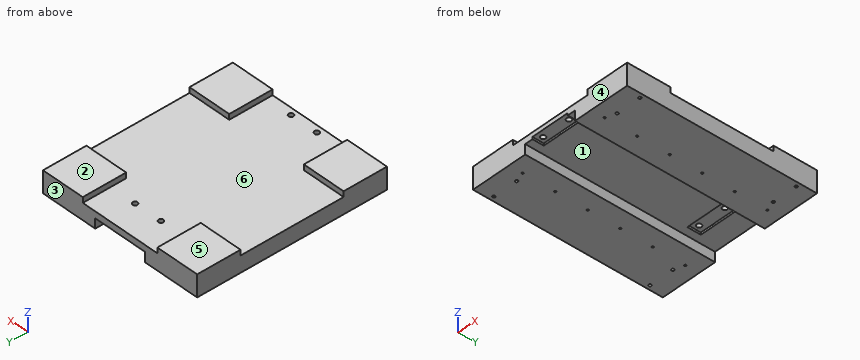
```python
from build123d import *

# Parameters (mm, degrees)
SKETCH_1_W                  = 310
SKETCH_1_H                  = 350
EXTRUDE_1_DEPTH             = 30
SKETCH_2_W                  = 100
SKETCH_2_H                  = 18
CUT_EXTRUDE_1_DEPTH         = 384.959633295
SKETCH_3_W                  = 80
SKETCH_3_H                  = 80
EXTRUDE_2_DEPTH             = 10
SKETCH_5_W                  = 71
SKETCH_5_H                  = 4
CUT_EXTRUDE_3_DEPTH         = 21
SKETCH_7_W                  = 71
SKETCH_7_H                  = 25
CUT_EXTRUDE_4_DEPTH         = 4
SKETCH_8_R                  = 4.5
CUT_EXTRUDE_5_DEPTH         = 235.806303152
HOLE_WIZARD_M6_1_D          = 5
HOLE_WIZARD_M6_1_DEPTH      = 12
HOLE_WIZARD_M6_1_TIP        = 1.502151548
HOLE_WIZARD_M4_1_AT_2_COUNT = 2
HOLE_WIZARD_M4_1_AT_2_PITCH = 165
PATTERN_LINEAR_1_COUNT      = 6
PATTERN_LINEAR_1_PITCH      = 60


with BuildPart() as part:
    # 草图1 → 凸台-拉伸1 (new body)
    with BuildSketch(Plane.XY):
        Rectangle(SKETCH_1_W, SKETCH_1_H)
    extrude(amount=EXTRUDE_1_DEPTH)

    # 草图2 → 切除-拉伸1 (cut, through all)
    with BuildSketch(Plane(origin=(0, 175, 0), x_dir=(1, 0, 0), z_dir=(0, 1, 0))):
        with Locations((0, -9)):
            Rectangle(SKETCH_2_W, SKETCH_2_H)
    extrude(amount=-CUT_EXTRUDE_1_DEPTH, mode=Mode.SUBTRACT)

    # 草图3 → 凸台-拉伸2 (add)
    with BuildSketch(Plane.XY.offset(30)):
        with Locations((-115, 135)):
            Rectangle(SKETCH_3_W, SKETCH_3_H)
        with Locations((115, 135)):
            Rectangle(SKETCH_3_W, SKETCH_3_H)
        with Locations((-115, -135)):
            Rectangle(SKETCH_3_W, SKETCH_3_H)
        with Locations((115, -135)):
            Rectangle(SKETCH_3_W, SKETCH_3_H)
    extrude(amount=EXTRUDE_2_DEPTH)

    # 草图5 → 切除-拉伸3 (cut)
    with BuildSketch(Plane.XZ.offset(175)):
        with Locations((0, 20)):
            Rectangle(SKETCH_5_W, SKETCH_5_H)
    extrude(amount=-CUT_EXTRUDE_3_DEPTH, mode=Mode.SUBTRACT)

    # 草图7 → 切除-拉伸4 (cut)
    with BuildSketch(Plane(origin=(0, 0, 18), x_dir=(-1, 0, 0), z_dir=(0, 0, -1))):
        with Locations((0, 123)):
            Rectangle(SKETCH_7_W, SKETCH_7_H)
    extrude(amount=-CUT_EXTRUDE_4_DEPTH, mode=Mode.SUBTRACT)

    # 草图8 → 切除-拉伸5 (cut, through all)
    with BuildSketch(Plane(origin=(0, 0, 18), x_dir=(-1, 0, 0), z_dir=(0, 0, -1))):
        with Locations((-26, 123.5)):
            Circle(SKETCH_8_R)
        with Locations((26, 123.5)):
            Circle(SKETCH_8_R)
        with Locations((-26, -164)):
            Circle(SKETCH_8_R)
        with Locations((26, -164)):
            Circle(SKETCH_8_R)
    extrude(amount=-CUT_EXTRUDE_5_DEPTH, mode=Mode.SUBTRACT)

    # M6 螺纹孔1
    with Locations(Plane(origin=(147, 144, 0), x_dir=(-1, 0, 0), z_dir=(0, 0, -1))):
        with Locations((0, 0), (46, 0), (248, 0), (294, 0), (0, -288), (46, -288), (248, -288), (294, -288)):
            Hole(HOLE_WIZARD_M6_1_D / 2, depth=HOLE_WIZARD_M6_1_DEPTH)
            with Locations((0, 0, -(HOLE_WIZARD_M6_1_DEPTH + HOLE_WIZARD_M6_1_TIP / 2))):  # 118° drill point
                Cone(0, HOLE_WIZARD_M6_1_D / 2, HOLE_WIZARD_M6_1_TIP, mode=Mode.SUBTRACT)

    # 草图14 → M4 螺纹孔1 (revolve, cut)
    with BuildSketch(Plane(origin=(82.5, 150, 0), x_dir=(0, 1, 0), z_dir=(1, 0, 0))):
        Polygon((0, 0), (0, 10.991420021), (1.65, 10), (1.65, 0), align=None)
    hole_wizard_m4_1 = revolve(axis=Axis((82.5, 150, -6.35), (0, 0, 1)), mode=Mode.SUBTRACT)

    # M4 螺纹孔1 at 2: M4 螺纹孔1 ×2
    with Locations(*[(-i * HOLE_WIZARD_M4_1_AT_2_PITCH, 0, 0) for i in range(1, HOLE_WIZARD_M4_1_AT_2_COUNT)]):
        add(hole_wizard_m4_1, mode=Mode.SUBTRACT)

    # 阵列(线性)1: M4 螺纹孔1 ×6
    with Locations(*[(0, -i * PATTERN_LINEAR_1_PITCH, 0) for i in range(1, PATTERN_LINEAR_1_COUNT)]):
        add(hole_wizard_m4_1, mode=Mode.SUBTRACT)

    # 阵列(线性)1 copy 1 sketch → 阵列(线性)1 copy 1 (revolve, cut)
    with BuildSketch(Plane(origin=(-82.5, 90, 0), x_dir=(0, 1, 0), z_dir=(1, 0, 0))):
        Polygon((0, 0), (0, 10.991420021), (1.65, 10), (1.65, 0), align=None)
    revolve(axis=Axis((-82.5, 90, -6.35), (0, 0, 1)), mode=Mode.SUBTRACT)

    # 阵列(线性)1 copy 2 sketch → 阵列(线性)1 copy 2 (revolve, cut)
    with BuildSketch(Plane(origin=(-82.5, 30, 0), x_dir=(0, 1, 0), z_dir=(1, 0, 0))):
        Polygon((0, 0), (0, 10.991420021), (1.65, 10), (1.65, 0), align=None)
    revolve(axis=Axis((-82.5, 30, -6.35), (0, 0, 1)), mode=Mode.SUBTRACT)

    # 阵列(线性)1 copy 3 sketch → 阵列(线性)1 copy 3 (revolve, cut)
    with BuildSketch(Plane(origin=(-82.5, -30, 0), x_dir=(0, 1, 0), z_dir=(1, 0, 0))):
        Polygon((0, 0), (0, 10.991420021), (1.65, 10), (1.65, 0), align=None)
    revolve(axis=Axis((-82.5, -30, -6.35), (0, 0, 1)), mode=Mode.SUBTRACT)

    # 阵列(线性)1 copy 4 sketch → 阵列(线性)1 copy 4 (revolve, cut)
    with BuildSketch(Plane(origin=(-82.5, -90, 0), x_dir=(0, 1, 0), z_dir=(1, 0, 0))):
        Polygon((0, 0), (0, 10.991420021), (1.65, 10), (1.65, 0), align=None)
    revolve(axis=Axis((-82.5, -90, -6.35), (0, 0, 1)), mode=Mode.SUBTRACT)

    # 阵列(线性)1 copy 5 sketch → 阵列(线性)1 copy 5 (revolve, cut)
    with BuildSketch(Plane(origin=(-82.5, -150, 0), x_dir=(0, 1, 0), z_dir=(1, 0, 0))):
        Polygon((0, 0), (0, 10.991420021), (1.65, 10), (1.65, 0), align=None)
    revolve(axis=Axis((-82.5, -150, -6.35), (0, 0, 1)), mode=Mode.SUBTRACT)


solid = part.part
```
The listing builds one solid part. Answer for the finished solid, in the listing's coordinates (mm). Face numbers are marked on the shaded views. A direction names the side the tool comes from. Give positions to 0.01 mm unless a question says otherwise; leave off trailing zeros. Write each loop counter-clockwise with the first axis right and the second up, starting at its lowest first coordinate (ties: lowest second). Pieces come first, ordered by that corner, then holes. Notation, with made-up numbers: (7, 65) - (51, 65) arc R17 ccw to (51, 94) - close; hole circle Ø3 at (14, 87.5). An arc over 180 degrees is marked (long way). Use one line per item in the form item = value. Start each with the question number.
1) Find section D-D on x = -112.5. Determine the outline of the cut face in (y, z).
2) Find section C-C on z = 34.5. Determine the outline of the cut face in (x, y).
3) Flat-ended cylindrical pins translate along their axes: pin 1 Ø1.5 at (x, y) = (-92.5, -20.5) entering from +Z; pin 2 Ø23 at (x, y) = (6, -163.5) entering from -Z; pin 3 Ø7.5 at (x, y) = (12.5, 119.5) entering from -Z; pin 4 Ø7 at (x, y) = (26, -164) entering from +Z. Find the tip coordinate at first contact, or state that the pin passes through.
4) A tool of negligible diameter and unlimited length cuts with its end or side. For the marked faces 1 and 2, from which of +Z, -Z, +X, -X, +Y, -Y can it reach the whole face along a straight path? Write none if from no direction.
5) Find section B-B on z = 4.5. Count the separate pieces of the cut face and the enclosed holes in it, plus the area to 3 significant figures.
6) The mould has two halves that part along Y. Classify the marked faces 3, 4, 5 and 6: pulls with the +Y half, pulls with the -Y half, needs draft (parallel to the pull), parting line crosses it, or undercut.
7) Find section A-A on y = 123.5. Determine the outline of the cut face in (x, z).
8) Consider line 1 along Y through (x, z) = (-26, 25); line 2 along X through (y, z) = (-150, 5.75); line 3 along Y through (x, z) = (-101, 3.25). Determine where each line is inside the solid, lowest interval first. Write a range as from..to.
Geometry results:
q1.outline = (-175, 0) - (175, 0) - (175, 40) - (95, 40) - (95, 30) - (-95, 30) - (-95, 40) - (-175, 40) - close
q2.outline = (-155, -175) - (-75, -175) - (-75, -95) - (-155, -95) - close; (-155, 95) - (-75, 95) - (-75, 175) - (-155, 175) - close; (75, -175) - (155, -175) - (155, -95) - (75, -95) - close; (75, 95) - (155, 95) - (155, 175) - (75, 175) - close
q3.pin_1 = 30
q3.pin_2 = 18
q3.pin_3 = 22
q3.pin_4 = through
q4.face_1 = -Z, +Y, -Y
q4.face_2 = +Z, +X, -X, +Y, -Y
q5.separate_pieces = 2
q5.enclosed_holes = 20
q5.area = 73,200 mm2
q6.face_3 = pulls with the +Y half
q6.face_4 = pulls with the -Y half
q6.face_5 = needs draft
q6.face_6 = undercut
q7.outline = (-155, 0) - (-50, 0) - (-50, 18) - (-35.5, 18) - (-35.5, 22) - (-30.5, 22) - (-30.5, 30) - (-75, 30) - (-75, 40) - (-155, 40) - close; (-21.5, 22) - (21.5, 22) - (21.5, 30) - (-21.5, 30) - close; (30.5, 22) - (35.5, 22) - (35.5, 18) - (50, 18) - (50, 0) - (155, 0) - (155, 40) - (75, 40) - (75, 30) - (30.5, 30) - close
q8.line_1 = -175..-168.5, -159.5..119, 128..175
q8.line_2 = -155..-84.15, -80.85..-50, 50..80.85, 84.15..155
q8.line_3 = -175..-146.5, -141.5..141.5, 146.5..175
